from build123d import *

# Parameters (mm, degrees)
F0_R     = 10.16
F1_DEPTH = 15.7734
F2_DEPTH = 40.2336
F3_R     = 3.302


with BuildPart() as f1:
    # F0 (on Top) → F1 (new body)
    with BuildSketch(Plane.XY):
        with BuildLine():
            Line((5.042647, -28.126541), (57.336765, -18.751028))
            ThreePointArc((57.336765, -18.751028), (73.025, 0), (57.336765, 18.751028))
            Line((57.336765, 18.751028), (5.042647, 28.126541))
            ThreePointArc((5.042647, 28.126541), (21.916025, 18.336262), (28.575, 0))
            ThreePointArc((28.575, 0), (21.916025, -18.336262), (5.042647, -28.126541))
        make_face()
        with Locations((53.975, 0)):
            Circle(F0_R, mode=Mode.SUBTRACT)
    extrude(amount=F1_DEPTH)

    # F0 (on Top) → F2 (join)
    with BuildSketch(Plane.XY):
        with BuildLine():
            ThreePointArc((5.042647, 28.126541), (-28.575, 0), (5.042647, -28.126541))
            ThreePointArc((5.042647, -28.126541), (21.916025, -18.336262), (28.575, 0))
            ThreePointArc((28.575, 0), (21.916025, 18.336262), (5.042647, 28.126541))
        make_face()
        with BuildLine():
            ThreePointArc((13.447765, -4.826), (-14.2875, 0), (13.447765, 4.826))
            Line((13.447765, 4.826), (18.527765, 4.826))
            Line((18.527765, 4.826), (18.527765, -4.826))
            Line((18.527765, -4.826), (13.447765, -4.826))
        make_face(mode=Mode.SUBTRACT)
    extrude(amount=F2_DEPTH)

    # F3
    f3_edges = [f1.edges().sort_by_distance(p)[0] for p in [
        (-5.042647, 28.126541, 40.2336),
    ]]
    fillet(f3_edges, radius=F3_R)


solid = f1.part
Build history of the part. All positions in model axes, mm. A direction names the side the tool comes from. Coordinates: 2 decimals unless noted, no trailing zeros. Write each loop counter-clockwise with the first axis right and the second up, starting at its lowest first coordinate (ties: lowest second). Pieces come first, ordered by that corner, then holes. Notation, with made-up numbers: (84.5, 79.5) -> (90.5, 79.5) arc R25 cw to (90.5, 112.5) -> close; hole circle Ø9 at (75, -23.75). An arc over 180 degrees is marked (long way). Use CSV: the item, a comma, the result in double quotes. Start each with the question number.
Q1. Cut at C-C, the plane x = 31. List the corners of the cut face in (y, z), then the cut area to 3 significant figures.
Q2. Drill centre lines: probe 1 along Y at (x, z) = (52.5, 6.5); probe 2 along Y at (x, z) = (-11.5, 3); probe 3 along X at (y, z) = (8, 14.5). Where is each one in solid material? Low to high.
Q3. Cut at B-B, the plane z = 8.5. State how many separate pieces and enclosed holes the cut face has, then the cut area to 3 significant figures.
Q4. 3-axis set-ups, long thin cutter, end or side, ignore diameter. For faces 1 (the flat face through (16, 4.826, 20)), 2 (the flat face through (22, 0, 0)): which of +Z, -Z, +X, -X, +Y, -Y reach the whole face in a straight line?
Q5. Flat gauge pins, fed straight in: pin 1 Ø1.5 at (y, z) = (5, 16) entering from +X; pin 2 Ø12 at (y, z) = (1.5, 9) entering from +X (3 decimals); pin 3 Ø4 at (x, z) = (15, 21.5) entering from +Y. Where does each tip first touch, or does it go through?
Q6. Pull direction X, two halves, no side cores. Call faces 3 (the flat face through (16, -4.826, 20)), 4 (the flat face through (30.824, -23.504, 7.776)), 5 (the cylindrical face through (-14.277, -0.559, 19.835)), 6 (the flat face through (11, -11, 40.234)): released by +X, released by -X, zero draft, split by the parting line, or undercut.
Checked values:
1,outline,"(-23.47, 0) -> (23.47, 0) -> (23.47, 15.77) -> (-23.47, 15.77) -> close"
1,area,"740 mm²"
2,probe 1,"y = -19.62 to -10.05, 10.05 to 19.62"
2,probe 2,"y = -26.16 to -8.48, 8.48 to 26.16"
2,probe 3,"x = -27.43 to -11.84, 11.84 to 47.71, 60.24 to 71.26"
3,separate pieces,"1"
3,enclosed holes,"2"
3,area,"3,450 mm²"
4,face 1,"+Z, -Z"
4,face 2,"-Z, +X, -X, +Y, -Y"
5,pin 1,"stops at x = 72.54"
5,pin 2,"stops at x = 73.025"
5,pin 3,"stops at y = 25.45"
6,face 3,"undercut"
6,face 4,"released by +X"
6,face 5,"undercut"
6,face 6,"zero draft"
